Work out the finished part from the listing and answer in its coordinate system (mm). A direction names the side the tool comes from. Give positions to 0.01 mm unless a question says otherwise; leave off trailing zeros. Loops run counter-clockwise (first coordinate to the right, second up) from the corner with the lowest first, then second, coordinate; pieces in that order, holes last. Notation, with made-up numbers: (14.5, 79.5) - (50.5, 79.5) arc R21 cw to (50.5, 110.5) - close; hole circle Ø6 at (65.5, 70). An arc over 180 degrees is marked (long way). One line per question, with ' | ' between items. Start each with the question number.
1. Find the intervals of material crossed by line 1 (X direction, y = -12.7, z = -8.5); line 2 (Y direction, x = 0, z = -8.5); line 3 (Z direction, x = -7, y = -16.5), in increasing order.
2. Section C-C (z = 7) is taken. Determine the outline of the cut face in (x, y), plus the area to 3 significant figures.
3. Section B-B (z = 0) is taken. Determine the outline of the cut face in (x, y).
4. For a pull along Y with two mould halves and no side action, classify faces 6 (the face through (0, -7.62, 0)), 7 (the face through (-12.7, -6.9, -3)), 8 (the face through (-4.68, -16.99, -8.94)), 9 (the face through (-4.68, -8.41, 8.94)) as released by +Y, released by -Y, zero draft, split by the parting line, or undercut.
5. Which of the six approach directions +Z, -Z, +X, -X, +Y, -Y give full straight-line access (tool end or side, diameter ignored) to faces 1 (the face through (0, -13, -5.08)), 2 (the face through (-5.08, -13, 0)), 3 (the face through (4.68, -3.76, 4.29)), 4 (the face through (5.08, -13, 0)), 5 (the face through (0, -13, 5.08))?
6. Section D-D (y = -1.75) is taken. Determine the outline of the cut face in (x, z).
7. Section A-A (y = -12.7) is taken. Determine the outline of the cut face in (x, z).
8. Each of these flat-tipped pins is pushed along its axis until it touches: pin 1 (11 mm diameter, centred on y = -12, z = 2, fed in from +X); pin 2 (3 mm diameter, centred on x = -1.5, z = -0.5, fed in from +Y); pin 3 (11.5 mm diameter, centred on y = -12.7, z = 0, fed in from -X); pin 4 (3 mm diameter, centred on x = 0.5, y = -14, fed in from -Z). Where does it stop, or does it pass through?
from build123d import *

# Parameters (mm, degrees)
F0_W      = 25.4
F0_H      = 25.4
F1_DEPTH  = 25.4
F2_R      = 6.35
F3_DEPTH  = 7.62
F4_R      = 6.35
F5_DEPTH  = 7.62
F6_R      = 6.35
F7_DEPTH  = 7.62
F8_R      = 6.35
F9_DEPTH  = 7.62
F10_R     = 6.35
F11_DEPTH = 7.62
F12_R     = 6.35
F13_DEPTH = 7.62


# Not quite as in the source:
# - a feature names something its author has since deleted; it is built from what else it names


with BuildPart() as f1:
    # F0 (on Front) → F1 (new body)
    with BuildSketch(Plane.XZ):
        Rectangle(F0_W, F0_H)
    extrude(amount=F1_DEPTH)

    # F2 (on face) → F3 (cut)
    with BuildSketch(Plane.XZ.offset(25.4)):
        Circle(F2_R)
    extrude(amount=-F3_DEPTH, mode=Mode.SUBTRACT)

    # F4 (on face) → F5 (cut)
    with BuildSketch(Plane(origin=(0, 0, 0), x_dir=(-1, 0, 0), z_dir=(0, 1, 0))):
        Circle(F4_R)
    extrude(amount=-F5_DEPTH, mode=Mode.SUBTRACT)

    # F6 (on face) → F7 (cut)
    with BuildSketch(Plane.YZ.offset(12.7)):
        with Locations((-12.7, 0)):
            Circle(F6_R)
    extrude(amount=-F7_DEPTH, mode=Mode.SUBTRACT)

    # F8 (on face) → F9 (cut)
    with BuildSketch(Plane(origin=(-12.7, 0, 0), x_dir=(0, -1, 0), z_dir=(-1, 0, 0))):
        with Locations((12.7, 0)):
            Circle(F8_R)
    extrude(amount=-F9_DEPTH, mode=Mode.SUBTRACT)

    # F10 (on face) → F11 (cut)
    with BuildSketch(Plane.XY.offset(12.7)):
        with Locations((0, -12.7)):
            Circle(F10_R)
    extrude(amount=-F11_DEPTH, mode=Mode.SUBTRACT)

    # F12 (on face) → F13 (cut)
    with BuildSketch(Plane(origin=(0, 0, -12.7), x_dir=(1, 0, 0), z_dir=(0, 0, -1))):
        with Locations((0, 12.7)):
            Circle(F12_R)
    extrude(amount=-F13_DEPTH, mode=Mode.SUBTRACT)


solid = f1.part
Conclusion:
1) line 1: -12.7 to -6.35, 6.35 to 12.7 | line 2: -25.4 to -19.05, -6.35 to 0 | line 3: -12.7 to -5.09, 5.09 to 12.7
2) outline: (-12.7, -25.4) - (12.7, -25.4) - (12.7, 0) - (-12.7, 0) - close; hole circle Ø12.7 at (0, -12.7) | area: 518 mm²
3) outline: (-12.7, -25.4) - (-6.35, -25.4) - (-6.35, -19.05) - (-12.7, -19.05) - close; (-12.7, -6.35) - (-6.35, -6.35) - (-6.35, 0) - (-12.7, 0) - close; (-5.08, -17.78) - (5.08, -17.78) - (5.08, -7.62) - (-5.08, -7.62) - close; (6.35, -25.4) - (12.7, -25.4) - (12.7, -19.05) - (6.35, -19.05) - close; (6.35, -6.35) - (12.7, -6.35) - (12.7, 0) - (6.35, 0) - close
4) face 6: released by +Y | face 7: zero draft | face 8: undercut | face 9: undercut
5) face 1: -Z | face 2: -X | face 3: +Y | face 4: +X | face 5: +Z
6) outline: (-12.7, -12.7) - (12.7, -12.7) - (12.7, 12.7) - (-12.7, 12.7) - close; hole circle Ø12.7 at (0, 0)
7) outline: (-12.7, -12.7) - (-6.35, -12.7) - (-6.35, -6.35) - (-12.7, -6.35) - close; (-12.7, 6.35) - (-6.35, 6.35) - (-6.35, 12.7) - (-12.7, 12.7) - close; (-5.08, -5.08) - (5.08, -5.08) - (5.08, 5.08) - (-5.08, 5.08) - close; (6.35, -12.7) - (12.7, -12.7) - (12.7, -6.35) - (6.35, -6.35) - close; (6.35, 6.35) - (12.7, 6.35) - (12.7, 12.7) - (6.35, 12.7) - close
8) pin 1: x = 12.7 | pin 2: y = -7.62 | pin 3: x = -5.08 | pin 4: z = -5.08
